Input: part model. Units: mm. Frame: model coordinates. A direction names the side the tool comes from. Coordinates: 2 decimals unless noted, no trailing zeros. Order: outer loops, then holes, each group sorted by start corner. A loop starts at its lowest first (then second) coordinate and runs counter-clockwise, first axis right, second up. Notation, with made-up numbers: (71, -1.5) -> (121, -1.5) arc R29 cw to (121, 26.5) -> close; hole circle Ø1 at (43.25, 26). An arc over 180 degrees is marked (long way). Use one line per item in the form item = value. Start each with the question number.
1) Draft query along Z for faces 1 (the flat face through (24, 42, -34.636)), 2 (the flat face through (24, 54.257, -17)), 3 (the cylindrical face through (20.801, 44.753, -6.524)). Return one class per face: pulls with the +Z half, pulls with the -Z half, needs draft (parallel to the pull), parting line crosses it, or undercut.
2) Section query C-C on y = 52. Output: boundary loops of the cut face in (x, z).
3) Section query B-B on x = 20.85. Output: boundary loops of the cut face in (y, z).
4) Section query A-A on z = -21. Output: boundary loops of the cut face in (x, y) (3 decimals).
5) Pin query (flat end, axial travel): pin 1 (3.5 mm diameter, centred on y = 41.5, z = -8, fed in from -X); pin 2 (1.5 mm diameter, centred on x = 21.5, y = 43.5, fed in from -Z); pin 3 (2.5 mm diameter, centred on y = 41.29, z = -7.01, fed in from -X). Return the tip coordinate at first contact, or that it passes through.
6) Access query for faces 4 (the cylindrical face through (20.801, 43.475, -6.726)), 5 (the flat face through (24, 29.725, -16)). Directions: +Z, -Z, +X, -X, +Y, -Y. A direction counts if a zero-diameter tool reaches every point of the face in a straight line with its end or side. Return the directions, or none.
7) Ray query, line 1 along X through (y, z) = (48.25, -13); line 2 along Z through (x, y) = (19.85, 44.5); line 3 along Y through (x, z) = (19.8, -19.5). Return the intervals inside material, ascending.
8) Section query D-D on x = 23.75. Output: boundary loops of the cut face in (y, z) (3 decimals), then the cut area to 3 significant figures.
Autodesk Inventor part; units mm, degrees
ref_plane "Work Plane1" through (25.2802, 41.8518, -22.309) normal (1, 0, 0) x (0, 1, 0)
ref_plane "YZ Plane" through (0, 0, 0) normal (1, 0, 0) x (0, 1, 0)
ref_plane "XZ Plane" through (0, 0, 0) normal (0, 1, 0) x (-1, 0, 0)
ref_plane "Work Plane1" through (25.2802, 41.8518, -22.309) normal (1, 0, 0) x (0, 1, 0)
sketch "Sketch1" plane through (25.2802, 41.8518, -22.309) normal (1, 0, 0) x (0, 1, 0)
  line L0 (12.4048, 23.6333) -> (-12.1268, 23.6333)
  line L1 (-12.1268, 23.6333) -> (-12.1268, -12.3269)
  line L2 (12.4048, -12.3269) -> (12.4048, 23.6333)
  line L3 (-12.1268, -12.3269) -> (12.4048, -12.3269)
  circle A0 centre (0, 0) radius 2.2
  circle A1 centre (-0.5578, 15.2966) radius 2.2
  line L4 (12.4048, 23.6333) -> (-12.1268, 23.6333)
  line L5 (-12.1268, 23.6333) -> (-12.1268, -12.3269)
  line L6 (-12.1268, -12.3269) -> (12.4048, -12.3269)
  line L7 (12.4048, -12.3269) -> (12.4048, 23.6333)
  circle A2 centre (-0.569, 15.3293) radius 3.5
  circle A3 centre (0, 0) radius 3.2587
  point P0 (-41.8518, 22.309)
extrude "Extrusion1" add sketch "Sketch1" against normal blind 3 contours L2 L3 L1 L0 | A1
sketch "Sketch2" plane through (25.2802, 41.8518, -22.309) normal (1, 0, 0) x (0, 0, -1)
  circle A0 centre (-15.2966, -0.5578) radius 2.2
  circle A1 centre (0, 0) radius 2.2
  circle A2 centre (-15.3293, -0.569) radius 3.5
  circle A3 centre (-15.3293, -0.569) radius 3.5
  circle A4 centre (0, 0) radius 3.2587
  point P0 (-22.309, -41.8518)
extrude "Extrusion2" add sketch "Sketch2" against normal blind 6
properties part number "GearBoxLid2"
Answers below:
q1.face_1 = pulls with the -Z half
q1.face_2 = needs draft
q1.face_3 = undercut
q2.outline = (22.28, -34.64) -> (25.28, -34.64) -> (25.28, 1.32) -> (22.28, 1.32) -> close
q3.outline = circle Ø7 at (41.28, -6.98); circle Ø6.52 at (41.85, -22.31); hole circle Ø4.4 at (41.29, -7.01); hole circle Ø4.4 at (41.85, -22.31)
q4.outline = (19.28, 38.868) -> (22.28, 38.868) -> (22.28, 29.725) -> (25.28, 29.725) -> (25.28, 40.084) -> (19.28, 40.084) -> close; (19.28, 43.62) -> (25.28, 43.62) -> (25.28, 54.257) -> (22.28, 54.257) -> (22.28, 44.836) -> (19.28, 44.836) -> close
q5.pin_1 = 19.28
q5.pin_2 = -25.44
q5.pin_3 = 22.28
q6.face_4 = -X
q6.face_5 = +Z, -Z, +X, -X, -Y
q7.line_1 = 22.28 to 25.28
q7.line_2 = -24.21 to -20.41, -8.36 to -5.6
q7.line_3 = 40.2 to 43.5
q8.outline = (29.725, -34.636) -> (54.257, -34.636) -> (54.257, 1.324) -> (29.725, 1.324) -> close; hole circle Ø4.4 at (41.852, -22.309)
q8.area = 867 mm^2
